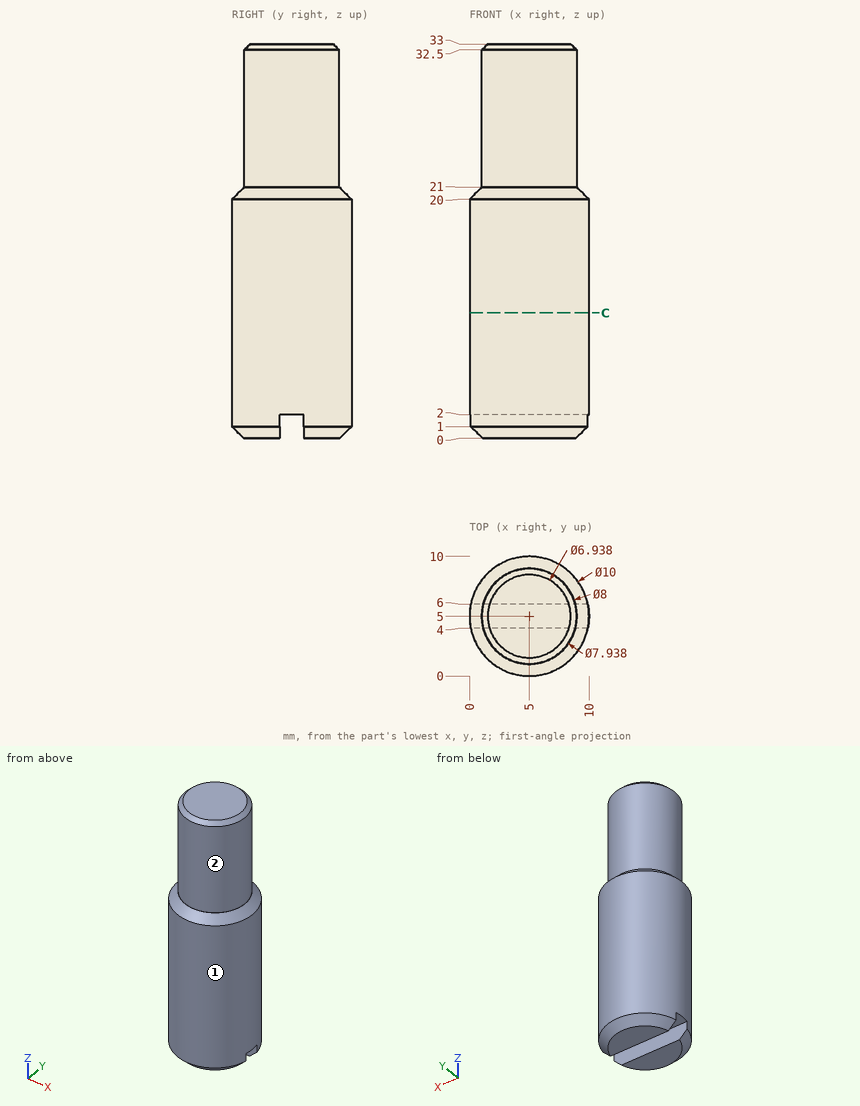
Can you work these out from the drawing? Everything is in mm from the part's minimum corner. A direction names the side the tool comes from. Coordinates: 2 decimals unless noted, no trailing zeros. Loops run counter-clockwise (first coordinate to the right, second up) from the corner with the lowest first, then second, coordinate; pieces in that order, holes last. Notation, with made-up numbers: (-5.75, 81.5) - (-0.75, 81.5) arc R24 ccw to (-0.75, 113.5) - close; hole circle Ø4 at (11.25, 85.25). An arc over 180 degrees is marked (long way). Put each result on its own line as item: value. Start each with the question number.
Item 1: Suppose I cut it at C-C (z = 10.5). Please give me the cut outline in (x, y).
Item 2: Which directions (+Z, -Z, +X, -X, +Y, -Y) give clear straight access to the entire face, cutting with the end or side of a thin tool? Please do the marked faces 1 and 2.
Item 3: For pin 1 (5 mm diameter, centred on x = 4, z = 27, fed in from +Y); pin 2 (3 mm diameter, centred on x = 8, z = 25.5, fed in from -Y) (1 decimal); pin 3 (6 mm diameter, centred on y = 8, z = 16, fed in from +X); pin 4 (2 mm diameter, centred on x = 3.5, z = 0.5, fed in from -Y), each with a flat end and sliding along its axis, tell me the tip position at first contact or that it passes through.
Item 4: If I drill on line 1 along X through (y, z) = (8, 10); line 2 along Z through (x, y) = (8, 6.75) (1 decimal); line 3 along X through (y, z) = (6, 17.5), over which ranges is the centre line in solid material (lowest first)?
Here are the results:
1. outline: circle Ø10 at (5, 5)
2. face 1: +Z, -Z
2. face 2: +Z
3. pin 1: y = 8.97
3. pin 2: y = 1.3
3. pin 3: x = 10
3. pin 4: y = 0.04
4. line 1: 1 to 9
4. line 2: 0 to 33
4. line 3: 0.1 to 9.9
